Verification items for the finished model (mm, model axes). A direction names the side the tool comes from. Give positions to 0.01 mm unless a question says otherwise; leave off trailing zeros. Loops run counter-clockwise (first coordinate to the right, second up) from the corner with the lowest first, then second, coordinate; pieces in that order, holes last. Notation, with made-up numbers: (0.25, 56) -> (19.25, 56) arc R21 cw to (19.25, 95) -> close; hole circle Ø5 at (71, 37.5). An arc over 180 degrees is marked (long way). Answer in a Markdown table with one row per item. Add a question column.
Q1. Set-up check for faces 4 (the face through (36, 5.357, -8)), 5 (the face through (7.76, -7.14, -21.66)), 6 (the face through (7.984, -5.297, 13.647)), 7 (the face through (36, -4.041, 15)): record each of +Z, -Z, +X, -X, +Y, -Y from which the full face is reachable in a straight line by a thin tool's end or side.
Q2. Section check C-C on z = -22. Enter the section's corners in (x, y), and give its area (3 significant figures).
Q3. Section check B-B on y = -10. Enter the section's corners in (x, z).
Q4. Section check A-A on x = 4.5. Enter the section's corners in (y, z).
Q5. Gauge pin test, flat ends, axial feed: P1, Ø3, axis at y = -11.5, z = -24.5, coming from the -X side; P2, Ø6.5, axis at x = 51, z = -6, coming from the +Y side; P3, Ø10.5, axis at x = 31, y = -1, coming from the -Z side; P4, Ø5, axis at x = 35.5, z = 25, coming from the -Y side. Record the tip position at first contact, or that the pin passes through.
Q6. Release check for a two-part mould opening along X. For faces 1 (the face through (57.404, -19, -12)), 2 (the face through (73.152, -8, 6)), 3 (the face through (36, 10, -1.34)) record: pulls with the +X half, pulls with the -X half, needs draft (parallel to the pull), parting line crosses it, or undercut.
Q7. Section check D-D on y = 8.5. Enter the section's corners in (x, z), and give its area (3 significant figures).
Q8. Material ranges on probe 1 along X at (y, z) = (8, 27.5); probe 2 along Y at (x, z) = (33.5, 35); probe 3 along X at (y, z) = (-16, -27), recorded low to high.
```python
from build123d import *

# Parameters (mm, degrees)
F1_DEPTH       = 73.152
F4_D           = 10.16
F4_CSINK_D     = 19.05
F4_CSINK_ANGLE = 82
F6_DEPTH       = 15.748
F7_R           = 6.3754
F8_DEPTH       = 15.748
F9_R           = 9.652


with BuildPart() as f1:
    # F0 (on Right) → F1 (new body)
    with BuildSketch(Plane.YZ):
        Polygon((15.0091618985, 43.1099530668), (-4.0408381015, 43.1099530668), (-4.0408381015, -14.0400469332), (5.3571618985, -14.0400469332), (5.3571618985, -1.3400469332), (15.0091618985, -1.3400469332), align=None)
    extrude(amount=F1_DEPTH)

    # F4 (through all)
    with Locations(Plane.XZ.offset(4.0408381015)):
        with Locations((17.526, 28.8859530668), (55.626, 28.8859530668)):
            CounterSinkHole(F4_D / 2, F4_CSINK_D / 2, counter_sink_angle=F4_CSINK_ANGLE)

    # F5 (on face) → F6 (join)
    with BuildSketch(Plane.YZ.offset(73.152)):
        with BuildLine():
            Line((-21.9497195355, -30.9575860672), (-2.432565009, -18.8660469332))
            Line((-2.432565009, -18.8660469332), (-15.2168381015, -18.8660469332))
            ThreePointArc((-15.2168381015, -18.8660469332), (-17.0135325512, -25.7858917839), (-21.9497195355, -30.9575860672))
        make_face()
        with BuildLine():
            Line((-29.4408381015, -4.6420469332), (-29.4408381015, -2.1335057937))
            Line((-29.4408381015, -2.1335057937), (-36.9319566675, -6.7745077991))
            ThreePointArc((-36.9319566675, -6.7745077991), (-33.3352009093, -5.1855456879), (-29.4408381015, -4.6420469332))
        make_face()
        with BuildLine():
            Line((-32.7984644588, -13.446446357), (-36.9319566675, -6.7745077991))
            ThreePointArc((-36.9319566675, -6.7745077991), (-41.5323772355, -26.3571654992), (-21.9497195355, -30.9575860672))
            Line((-21.9497195355, -30.9575860672), (-26.0832117442, -24.2856475093))
            ThreePointArc((-26.0832117442, -24.2856475093), (-34.8604386776, -22.2236732904), (-32.7984644588, -13.446446357))
        make_face()
        with BuildLine():
            ThreePointArc((-21.9497195355, -30.9575860672), (-17.0135325512, -25.7858917839), (-15.2168381015, -18.8660469332))
            Line((-15.2168381015, -18.8660469332), (-23.0654381015, -18.8660469332))
            ThreePointArc((-23.0654381015, -18.8660469332), (-23.8707422209, -21.9676202502), (-26.0832117442, -24.2856475093))
            Line((-26.0832117442, -24.2856475093), (-21.9497195355, -30.9575860672))
        make_face()
        with BuildLine():
            Line((-29.4408381015, -12.4906469332), (-29.4408381015, -4.6420469332))
            ThreePointArc((-29.4408381015, -4.6420469332), (-33.3352009093, -5.1855456879), (-36.9319566675, -6.7745077991))
            Line((-36.9319566675, -6.7745077991), (-32.7984644588, -13.446446357))
            ThreePointArc((-32.7984644588, -13.446446357), (-31.1863471457, -12.7342508393), (-29.4408381015, -12.4906469332))
        make_face()
        with BuildLine():
            Line((-4.0408381015, -14.0400469332), (-4.0408381015, 13.602655622))
            Line((-4.0408381015, 13.602655622), (-29.4408381015, -2.1335057937))
            Line((-29.4408381015, -2.1335057937), (-29.4408381015, -4.6420469332))
            ThreePointArc((-29.4408381015, -4.6420469332), (-19.3829512459, -8.8081600776), (-15.2168381015, -18.8660469332))
            Line((-15.2168381015, -18.8660469332), (-2.432565009, -18.8660469332))
            Line((-2.432565009, -18.8660469332), (5.3571618985, -14.0400469332))
            Line((5.3571618985, -14.0400469332), (-4.0408381015, -14.0400469332))
        make_face()
        with BuildLine():
            ThreePointArc((-15.2168381015, -18.8660469332), (-19.3829512459, -8.8081600776), (-29.4408381015, -4.6420469332))
            Line((-29.4408381015, -4.6420469332), (-29.4408381015, -12.4906469332))
            ThreePointArc((-29.4408381015, -12.4906469332), (-24.9327495287, -14.3579583604), (-23.0654381015, -18.8660469332))
            Line((-23.0654381015, -18.8660469332), (-15.2168381015, -18.8660469332))
        make_face()
    extrude(amount=-F6_DEPTH)

    # F7 (on face) → F8 (join)
    with BuildSketch(Plane(origin=(0, 0, 0), x_dir=(0, -1, 0), z_dir=(-1, 0, 0))):
        with BuildLine():
            ThreePointArc((19.9829674828, -29.4901167446), (35.2629264004, -31.8439305757), (43.6648381015, -18.8660469332))
            ThreePointArc((43.6648381015, -18.8660469332), (42.6255838026, -13.5289450231), (39.6596838836, -8.9717371097))
            Line((39.6596838836, -8.9717371097), (33.7111787045, -5.2982038056))
            ThreePointArc((33.7111787045, -5.2982038056), (17.0699133249, -11.8459047572), (19.9829674828, -29.4901167446))
        make_face()
        with Locations((29.4408381015, -18.8660469332)):
            Circle(F7_R, mode=Mode.SUBTRACT)
        with BuildLine():
            Line((-5.3571618985, -14.0400469332), (19.9829674828, -29.4901167446))
            ThreePointArc((19.9829674828, -29.4901167446), (17.0699133249, -11.8459047572), (33.7111787045, -5.2982038056))
            Line((33.7111787045, -5.2982038056), (4.0408381015, 13.0248842761))
            Line((4.0408381015, 13.0248842761), (4.0408381015, -14.0400469332))
            Line((4.0408381015, -14.0400469332), (-5.3571618985, -14.0400469332))
        make_face()
    extrude(amount=-F8_DEPTH)

    # F9
    f9_edges = [f1.edges().sort_by_distance(p)[0] for p in [
        (65.278, -4.040838, 13.602656),
        (7.874, -4.040838, 13.024884),
    ]]
    fillet(f9_edges, radius=F9_R)


solid = f1.part
```
Taken from the geometry:
| question | item | result |
|---|---|---|
| 1 | face 4 | -Z, +X, -X, +Y |
| 1 | face 5 | -Z, -X, +Y |
| 1 | face 6 | +Z, -X, -Y |
| 1 | face 7 | +Z, -Y |
| 2 | outline | (0, -43.32) -> (15.75, -43.32) -> (15.75, -34.99) -> (0, -34.99) -> close; (0, -23.89) -> (15.75, -23.89) -> (15.75, -7.7) -> (0, -7.7) -> close; (57.4, -43.32) -> (73.15, -43.32) -> (73.15, -34.99) -> (57.4, -34.99) -> close; (57.4, -23.89) -> (73.15, -23.89) -> (73.15, -7.49) -> (57.4, -7.49) -> close |
| 2 | area | 775 mm² |
| 3 | outline | (0, -23.4) -> (15.75, -23.4) -> (15.75, 9.34) -> (0, 9.34) -> close; (57.4, -23.55) -> (73.15, -23.55) -> (73.15, 9.91) -> (57.4, 9.91) -> close |
| 4 | outline | (-39.66, -8.97) arc R14.22 ccw to (-19.98, -29.49) -> (5.36, -14.04) -> (5.36, -1.34) -> (15.01, -1.34) -> (15.01, 43.11) -> (-4.04, 43.11) -> (-4.04, 18.41) arc R9.65 cw to (-8.62, 10.2) -> close; hole circle Ø12.75 at (-29.44, -18.87) |
| 5 | P1 | stops at x = 0 |
| 5 | P2 | stops at y = 5.36 |
| 5 | P3 | stops at z = -14.04 |
| 5 | P4 | stops at y = -4.04 |
| 6 | face 1 | undercut |
| 6 | face 2 | pulls with the +X half |
| 6 | face 3 | needs draft |
| 7 | outline | (0, -1.34) -> (73.15, -1.34) -> (73.15, 43.11) -> (0, 43.11) -> close; hole circle Ø10.16 at (17.53, 28.89); hole circle Ø10.16 at (55.63, 28.89) |
| 7 | area | 3,090 mm² |
| 8 | probe 1 | x = 0 to 12.64, 22.41 to 50.74, 60.51 to 73.15 |
| 8 | probe 2 | y = -4.04 to 15.01 |
| 8 | probe 3 | x = 0 to 15.75, 57.4 to 73.15 |
